Read the model definition and answer for the solid it produces. Units are mm, in the model's axes. Face numbers are marked on the shaded views. A direction names the side the tool comes from. Give positions to 0.01 mm unless a question says otherwise; leave off trailing zeros. Order: outer loops, then holes, each group sorted by start corner. A loop starts at its lowest first (then second) coordinate and runs counter-clockwise, first axis right, second up. Notation, with made-up numbers: (11.25, 31.5) - (16.25, 31.5) arc R18 ccw to (16.25, 57.5) - close; hole circle Ø11 at (76, 79.25). An arc over 180 degrees is marked (long way). Return JSON: item names as keys, results as strings.
```python
from build123d import *

# Parameters (mm, degrees)
SKETCH1_R           = 12
SKETCH1_R_2         = 2.1
BOSS_EXTRUDE1_DEPTH = 4
CUT_EXTRUDE1_DEPTH  = 3
CUT_EXTRUDE2_DEPTH  = 4
CIRPATTERN1_COUNT   = 8


with BuildPart() as part:
    # Sketch1 → Boss-Extrude1 (new body)
    with BuildSketch(Plane.XY):
        Circle(SKETCH1_R)
        Circle(SKETCH1_R_2, mode=Mode.SUBTRACT)
    extrude(amount=BOSS_EXTRUDE1_DEPTH)

    # Sketch2 → Cut-Extrude1 (cut)
    with BuildSketch(Plane.XY.offset(4)):
        Polygon((4.156921938, 0), (2.078460969, 3.6), (-2.078460969, 3.6), (-4.156921938, 0), (-2.078460969, -3.6), (2.078460969, -3.6), align=None)
    extrude(amount=-CUT_EXTRUDE1_DEPTH, mode=Mode.SUBTRACT)

    # Sketch3 → Cut-Extrude2 (cut)
    with BuildSketch(Plane.XY.offset(4)):
        Polygon((9.968896423, 2), (12.968896423, 4), (12.968896423, -4), (9.968896423, -2), align=None)
    cut_extrude2 = extrude(amount=-CUT_EXTRUDE2_DEPTH, mode=Mode.SUBTRACT)

    # CirPattern1: Cut-Extrude2 ×8 about axis
    cirpattern1_axis = Axis((0, 0, 0), (0, 0, 1))
    for i in range(1, CIRPATTERN1_COUNT):
        add(cut_extrude2.rotate(cirpattern1_axis, i * 360 / CIRPATTERN1_COUNT), mode=Mode.SUBTRACT)


solid = part.part
```
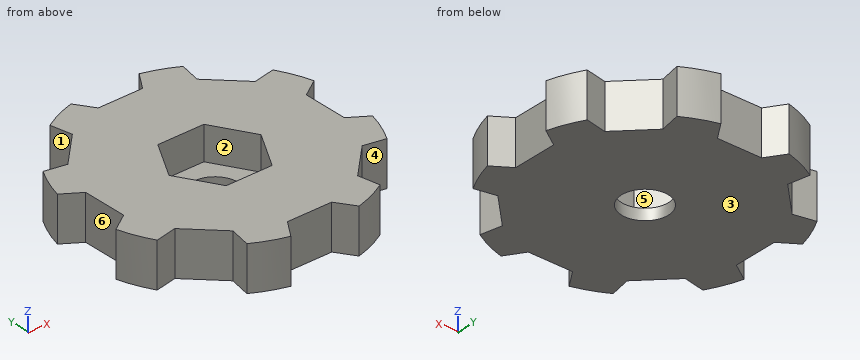
Q1. Determine the mould class of the marked faces 1, 2 and 3 for opening direction X: released by +X, released by -X, zero draft, split by the parting line, or undercut.
Values:
{"face 1": "released by -X", "face 2": "undercut", "face 3": "zero draft"}
Q2. A cutting plane is placed at A-A (x = 0). Write down the section's boundary in (y, z), and give its area (3 significant figures).
Values:
{"outline": "(-9.97, 0) - (-2.1, 0) - (-2.1, 1) - (-3.6, 1) - (-3.6, 4) - (-9.97, 4) - close; (2.1, 0) - (9.97, 0) - (9.97, 4) - (3.6, 4) - (3.6, 1) - (2.1, 1) - close", "area": "54.0 mm²"}
Q3. For the marked faces 4, 5 and 6, determine the directions among +Z, -Z, +X, -X, +Y, -Y from which every point of the face is accessible in a straight line to the end or side of a thin tool.
Values:
{"face 4": "+Z, -Z, -Y", "face 5": "+Z", "face 6": "+Z, -Z, -X"}
Q4. Given pin 1 (0.9 mm diameter, centred on x = 1, z = 2, fed in from +Y); pin 2 (1.5 mm diameter, centred on y = -0.5, z = 0.5, fed in from +X); pin 3 (1.5 mm diameter, centred on x = -0.5, z = 2.5, fed in from -Y), each flat-ended and moving along its own axis, determine where each tip first touches the part or whether it passes through.
Values:
{"pin 1": "stops at y = 9.97", "pin 2": "stops at x = 9.97", "pin 3": "stops at y = -9.97"}
Q5. Consider L1, parallel to Y at x = 0, z = 0.65; L2, parallel to Y at x = -1.5, z = 3.5. Determine where each line is inside the solid, lowest interval first.
Values:
{"L1": "y = -9.97 to -2.1, 2.1 to 9.97", "L2": "y = -9.97 to -3.6, 3.6 to 9.97"}
